Work out the finished part from the listing and answer in its coordinate system (mm). A direction names the side the tool comes from. Give positions to 0.01 mm unless a question says otherwise; leave off trailing zeros. Write each loop counter-clockwise with the first axis right and the second up, starting at its lowest first coordinate (ties: lowest second). Pieces come first, ordered by that corner, then holes.
1) A tool of negligible diameter and unlimited length cuts with its end or side. For faces 4 (the face through (-11.12, -3.13, 4.74)), 5 (the face through (4.694, -3.131, -11.067)), 6 (the face through (-2.46, -3.13, 9.2)), 7 (the face through (-7.237, -3.131, -9.599)), 8 (the face through (11.93, -3.13, -1.47)), from which of +Z, -Z, +X, -X, +Y, -Y can it reach the whole face along a straight path? Write none if from no direction.
2) Given pin 1 Ø1.5 at (y, z) = (-2, -9.5) entering from -X, flat-ended and moving along its own axis, determine where the tip first touches the part or whether it passes through.
3) Straight lines are drawn through the part: probe 1 along X at (y, z) = (-1.5, -11.5); probe 2 along Z at (x, y) = (0, -1.75) (1 decimal); probe 3 along Z at (x, y) = (-12.5, -0.75). For each, find the intervals that lie inside material, in ascending order.
4) Determine the mould class of faces 1 (the face through (-7.315, -3.131, -12.641)), 2 (the face through (2.47, -3.13, 9.2)), 3 (the face through (-7.263, -3.131, 9.669)) for opening direction Z: pulls with the +Z half, pulls with the -Z half, needs draft (parallel to the pull), parting line crosses it, or undercut.
5) Find section D-D (x = 4.75). Determine the outline of the cut face in (y, z), plus the area to 3 significant figures.
6) Find section C-C (x = 12.5). Determine the outline of the cut face in (y, z), plus the area to 3 significant figures.
```python
from build123d import *

# Parameters (mm, degrees)
F1_DEPTH = 6.35
F2_R     = 1.5875
F3_DEPTH = 6.35


with BuildPart() as f1:
    # F0 (on Front) → F1 (new body)
    with BuildSketch(Plane.XZ):
        with BuildLine():
            ThreePointArc((-6.318335, 7.127711), (-4.7625, 8.248892), (-3.013611, 9.035694))
            Line((-3.013611, 9.035694), (-6.422618, 13.156301))
            Line((-6.422618, 13.156301), (-7.3025, 12.648301))
            Line((-7.3025, 12.648301), (-8.182382, 12.140301))
            Line((-8.182382, 12.140301), (-6.318335, 7.127711))
        make_face()
        with BuildLine():
            ThreePointArc((-9.035694, 3.013611), (-8.248892, 4.7625), (-7.127711, 6.318335))
            Line((-7.127711, 6.318335), (-12.140301, 8.182382))
            Line((-12.140301, 8.182382), (-12.648301, 7.3025))
            Line((-12.648301, 7.3025), (-13.156301, 6.422618))
            Line((-13.156301, 6.422618), (-9.035694, 3.013611))
        make_face()
        with BuildLine():
            Line((-14.605, -1.016), (-9.331946, -1.907983))
            ThreePointArc((-9.331946, -1.907983), (-9.525, 0), (-9.331946, 1.907983))
            Line((-9.331946, 1.907983), (-14.605, 1.016))
            Line((-14.605, 1.016), (-14.605, 0))
            Line((-14.605, 0), (-14.605, -1.016))
        make_face()
        with BuildLine():
            Line((-6.422618, -13.156301), (-3.013611, -9.035694))
            ThreePointArc((-3.013611, -9.035694), (-4.7625, -8.248892), (-6.318335, -7.127711))
            Line((-6.318335, -7.127711), (-8.182382, -12.140301))
            Line((-8.182382, -12.140301), (-7.3025, -12.648301))
            Line((-7.3025, -12.648301), (-6.422618, -13.156301))
        make_face()
        with BuildLine():
            Line((-12.140301, -8.182382), (-7.127711, -6.318335))
            ThreePointArc((-7.127711, -6.318335), (-8.248892, -4.7625), (-9.035694, -3.013611))
            Line((-9.035694, -3.013611), (-13.156301, -6.422618))
            Line((-13.156301, -6.422618), (-12.648301, -7.3025))
            Line((-12.648301, -7.3025), (-12.140301, -8.182382))
        make_face()
        with BuildLine():
            ThreePointArc((9.331946, -1.907983), (9.476614, -0.958863), (9.525, 0))
            ThreePointArc((9.525, 0), (9.476614, 0.958863), (9.331946, 1.907983))
            ThreePointArc((9.331946, 1.907983), (9.200443, 2.465251), (9.035694, 3.013611))
            ThreePointArc((9.035694, 3.013611), (8.248892, 4.7625), (7.127711, 6.318335))
            ThreePointArc((7.127711, 6.318335), (6.735192, 6.735192), (6.318335, 7.127711))
            ThreePointArc((6.318335, 7.127711), (4.7625, 8.248892), (3.013611, 9.035694))
            ThreePointArc((3.013611, 9.035694), (2.465251, 9.200443), (1.907983, 9.331946))
            ThreePointArc((1.907983, 9.331946), (0.958863, 9.476614), (0, 9.525))
            ThreePointArc((0, 9.525), (-0.958863, 9.476614), (-1.907983, 9.331946))
            ThreePointArc((-1.907983, 9.331946), (-2.465251, 9.200443), (-3.013611, 9.035694))
            ThreePointArc((-3.013611, 9.035694), (-4.7625, 8.248892), (-6.318335, 7.127711))
            ThreePointArc((-6.318335, 7.127711), (-6.735192, 6.735192), (-7.127711, 6.318335))
            ThreePointArc((-7.127711, 6.318335), (-8.248892, 4.7625), (-9.035694, 3.013611))
            ThreePointArc((-9.035694, 3.013611), (-9.200443, 2.465251), (-9.331946, 1.907983))
            ThreePointArc((-9.331946, 1.907983), (-9.525, 0), (-9.331946, -1.907983))
            ThreePointArc((-9.331946, -1.907983), (-9.200443, -2.465251), (-9.035694, -3.013611))
            ThreePointArc((-9.035694, -3.013611), (-8.248892, -4.7625), (-7.127711, -6.318335))
            ThreePointArc((-7.127711, -6.318335), (-6.735192, -6.735192), (-6.318335, -7.127711))
            ThreePointArc((-6.318335, -7.127711), (-4.7625, -8.248892), (-3.013611, -9.035694))
            ThreePointArc((-3.013611, -9.035694), (-2.465251, -9.200443), (-1.907983, -9.331946))
            ThreePointArc((-1.907983, -9.331946), (0, -9.525), (1.907983, -9.331946))
            ThreePointArc((1.907983, -9.331946), (2.465251, -9.200443), (3.013611, -9.035694))
            ThreePointArc((3.013611, -9.035694), (4.7625, -8.248892), (6.318335, -7.127711))
            ThreePointArc((6.318335, -7.127711), (6.735192, -6.735192), (7.127711, -6.318335))
            ThreePointArc((7.127711, -6.318335), (8.248892, -4.7625), (9.035694, -3.013611))
            ThreePointArc((9.035694, -3.013611), (9.200443, -2.465251), (9.331946, -1.907983))
        make_face()
        with BuildLine():
            Line((1.016, -14.605), (1.907983, -9.331946))
            ThreePointArc((1.907983, -9.331946), (0, -9.525), (-1.907983, -9.331946))
            Line((-1.907983, -9.331946), (-1.016, -14.605))
            Line((-1.016, -14.605), (0, -14.605))
            Line((0, -14.605), (1.016, -14.605))
        make_face()
        with BuildLine():
            Line((8.182382, -12.140301), (6.318335, -7.127711))
            ThreePointArc((6.318335, -7.127711), (4.7625, -8.248892), (3.013611, -9.035694))
            Line((3.013611, -9.035694), (6.422618, -13.156301))
            Line((6.422618, -13.156301), (7.3025, -12.648301))
            Line((7.3025, -12.648301), (8.182382, -12.140301))
        make_face()
        with BuildLine():
            Line((13.156301, -6.422618), (9.035694, -3.013611))
            ThreePointArc((9.035694, -3.013611), (8.248892, -4.7625), (7.127711, -6.318335))
            Line((7.127711, -6.318335), (12.140301, -8.182382))
            Line((12.140301, -8.182382), (12.648301, -7.3025))
            Line((12.648301, -7.3025), (13.156301, -6.422618))
        make_face()
        with BuildLine():
            ThreePointArc((9.331946, 1.907983), (9.476614, 0.958863), (9.525, 0))
            ThreePointArc((9.525, 0), (9.476614, -0.958863), (9.331946, -1.907983))
            Line((9.331946, -1.907983), (14.605, -1.016))
            Line((14.605, -1.016), (14.605, 0))
            Line((14.605, 0), (14.605, 1.016))
            Line((14.605, 1.016), (9.331946, 1.907983))
        make_face()
        with BuildLine():
            ThreePointArc((7.127711, 6.318335), (8.248892, 4.7625), (9.035694, 3.013611))
            Line((9.035694, 3.013611), (13.156301, 6.422618))
            Line((13.156301, 6.422618), (12.648301, 7.3025))
            Line((12.648301, 7.3025), (12.140301, 8.182382))
            Line((12.140301, 8.182382), (7.127711, 6.318335))
        make_face()
        with BuildLine():
            ThreePointArc((3.013611, 9.035694), (4.7625, 8.248892), (6.318335, 7.127711))
            Line((6.318335, 7.127711), (8.182382, 12.140301))
            Line((8.182382, 12.140301), (7.3025, 12.648301))
            Line((7.3025, 12.648301), (6.422618, 13.156301))
            Line((6.422618, 13.156301), (3.013611, 9.035694))
        make_face()
        with BuildLine():
            ThreePointArc((-1.907983, 9.331946), (-0.958863, 9.476614), (0, 9.525))
            Line((0, 9.525), (0, 14.605))
            Line((0, 14.605), (-1.016, 14.605))
            Line((-1.016, 14.605), (-1.907983, 9.331946))
        make_face()
        with BuildLine():
            ThreePointArc((0, 9.525), (0.958863, 9.476614), (1.907983, 9.331946))
            Line((1.907983, 9.331946), (1.016, 14.605))
            Line((1.016, 14.605), (0, 14.605))
            Line((0, 14.605), (0, 9.525))
        make_face()
    extrude(amount=F1_DEPTH)

    # F2 (on face) → F3 (cut)
    with BuildSketch(Plane.XZ.offset(6.35)):
        Circle(F2_R)
    extrude(amount=-F3_DEPTH, mode=Mode.SUBTRACT)


solid = f1.part
```
Results:
1. face 4: -X, +Y, -Y
1. face 5: -Z, +Y, -Y
1. face 6: +Z, +Y, -Y
1. face 7: +Y, -Y
1. face 8: +X, +Y, -Y
2. pin 1: stops at x = -7.48
3. probe 1: x = -7.94 to -5.05, -1.54 to 1.54, 5.05 to 7.94
3. probe 2: z = -14.6 to -1.6, 1.6 to 14.6
3. probe 3: z = -7.56 to -5.88, -1.37 to 1.37, 5.88 to 7.56
4. face 1: pulls with the -Z half
4. face 2: pulls with the +Z half
4. face 3: undercut
5. outline: (-6.35, -11.13) - (0, -11.13) - (0, 11.13) - (-6.35, 11.13) - close
5. area: 141 mm2
6. outline: (-6.35, -7.56) - (0, -7.56) - (0, -5.88) - (-6.35, -5.88) - close; (-6.35, -1.37) - (0, -1.37) - (0, 1.37) - (-6.35, 1.37) - close; (-6.35, 5.88) - (0, 5.88) - (0, 7.56) - (-6.35, 7.56) - close
6. area: 38.8 mm2
